Geometry: see drawing. Coordinates: mm, zero at the bounding-box minimum. A direction names the side the tool comes from. Give positions to 0.01 mm unless a question says otherwise; leave off trailing zeros. Loops run counter-clockwise (first coordinate to the right, second up) from the corner with the lowest first, then second, coordinate; pieces in that order, holes last. Notation, with made-up numbers: (4.5, 62) -> (23.5, 62) arc R37 cw to (23.5, 99) -> close; hole circle Ø2 at (20.5, 86). An arc over 180 degrees is marked (long way). Return JSON: item names as keys, results as strings. Group by question number.
(1) Access query for the marked faces 1 and 2. Directions: +Z, -Z, +X, -X, +Y, -Y. A direction counts if a zero-diameter tool reaches every point of the face in a straight line with its end or side. Return the directions, or none.
(2) Pin query (flat end, axial travel): pin 1 (13 mm diameter, centred on x = 22.5, z = 18, fed in from -Y); pin 2 (8 mm diameter, centred on x = 55.5, y = 34.5, fed in from +Z). Return the tip coordinate at first contact, or that it passes through.
(3) Cut plane B-B on z = 35. Return loops of the section in (x, y), then the cut area to 3 significant figures.
(4) Ray query, line 1 (X direction, y = 46, z = 35); line 2 (Y direction, x = 6, z = 3.1); line 3 (Z direction, x = 61, y = 47). Return the intervals inside material, ascending. Write a range as from..to.
(5) Draft query along X for the marked faces 3 and 4. Return one class per face: released by +X, released by -X, zero draft, split by the parting line, or undercut.
(6) Cut plane C-C on y = 45. Return loops of the section in (x, z), then the cut area to 3 significant figures.
(7) Cut plane A-A on y = 26. Return loops of the section in (x, z).
(8) Cut plane D-D on x = 6.5. Return loops of the section in (y, z).
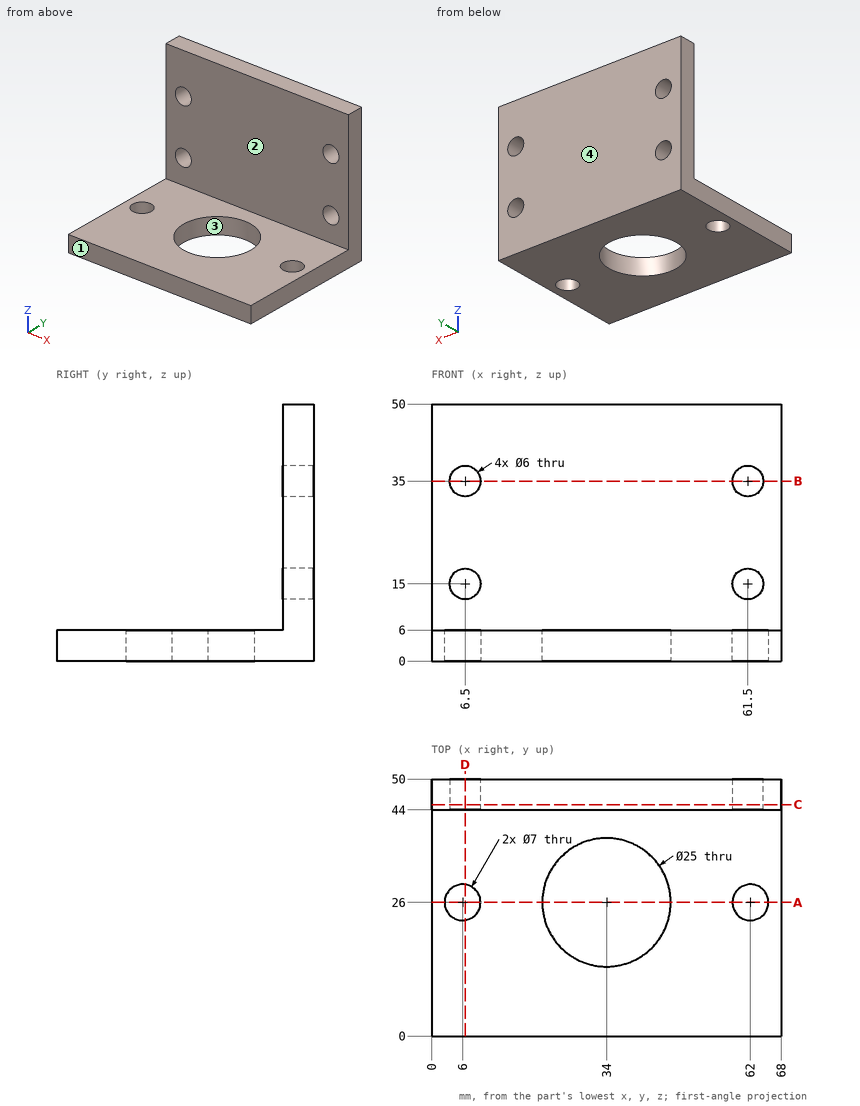
Answers:
{
 "1": {"face 1": "+Z, -Z, +X, -X, -Y", "face 2": "+Z, +X, -X, -Y"},
 "2": {"pin 1": "y = 44", "pin 2": "z = 6"},
 "3": {"outline": "(0, 44) -> (3.5, 44) -> (3.5, 50) -> (0, 50) -> close; (9.5, 44) -> (58.5, 44) -> (58.5, 50) -> (9.5, 50) -> close; (64.5, 44) -> (68, 44) -> (68, 50) -> (64.5, 50) -> close", "area": "336 mm²"},
 "4": {"line 1": "0..3.5, 9.5..58.5, 64.5..68", "line 2": "0..22.5, 29.5..50", "line 3": "0..12.04, 17.96..32.04, 37.96..50"},
 "5": {"face 3": "undercut", "face 4": "zero draft"},
 "6": {"outline": "(0, 0) -> (68, 0) -> (68, 50) -> (0, 50) -> close; hole circle Ø6 at (6.5, 15); hole circle Ø6 at (6.5, 35); hole circle Ø6 at (61.5, 15); hole circle Ø6 at (61.5, 35)", "area": "3,290 mm²"},
 "7": {"outline": "(0, 0) -> (2.5, 0) -> (2.5, 6) -> (0, 6) -> close; (9.5, 0) -> (21.5, 0) -> (21.5, 6) -> (9.5, 6) -> close; (46.5, 0) -> (58.5, 0) -> (58.5, 6) -> (46.5, 6) -> close; (65.5, 0) -> (68, 0) -> (68, 6) -> (65.5, 6) -> close"},
 "8": {"outline": "(0, 0) -> (22.54, 0) -> (22.54, 6) -> (0, 6) -> close; (29.46, 0) -> (50, 0) -> (50, 12) -> (44, 12) -> (44, 6) -> (29.46, 6) -> close; (44, 18) -> (50, 18) -> (50, 32) -> (44, 32) -> close; (44, 38) -> (50, 38) -> (50, 50) -> (44, 50) -> close"}
}
